Build history of the part. All positions in model axes, mm. Give positions to 0.01 mm unless a question says otherwise; leave off trailing zeros. Write each loop counter-clockwise with the first axis right and the second up, starting at its lowest first coordinate (ties: lowest second). Pieces come first, ordered by that corner, then holes. Notation, with made-up numbers: (-10, -8) -> (36, -8) arc R20 cw to (36, 16) -> close; hole circle Ø6 at (64.25, 70). An arc over 180 degrees is marked (long way). Write item = value, one per line. Start each with the question number.
Q1. Saw through at B-B, the plane y = 92.65. Give the number of separate pieces and of enclosed holes in the cut face, then the cut area to 3 significant figures.
Q2. Wall check: line 1 (X direction, y = 91.65, z = -6); line 2 (X direction, y = 92.9, z = -136.5); line 3 (X direction, y = 92.75, z = -112). Give the ranges that are in metal, low to high.
Q3. Drop a flat-ended pin along its axis: P1, Ø5, axis at x = 117, z = -6, coming from the +Y side. Give the stop position or say it passes through.
Q4. Saw through at A-A, the plane z = -21.5. List the corners of the cut face in (x, y), then the cut area to 3 significant figures.
from build123d import *

# Parameters (mm, degrees)
SKETCH1_W           = 123
SKETCH1_H           = 220
BOSS_EXTRUDE1_DEPTH = 4
SKETCH2_W           = 123
SKETCH2_H           = 220
SKETCH2_W_2         = 115
SKETCH2_H_2         = 212
BOSS_EXTRUDE2_DEPTH = 87
CUT_EXTRUDE1_REACH  = 269.974
SKETCH3_W           = 115
SKETCH3_H           = 45
CUT_EXTRUDE2_REACH  = 269.974
SKETCH4_W           = 150
SKETCH4_H           = 20
SKETCH6_W           = 24
SKETCH6_H           = 37
SKETCH6_R           = 1.45
BOSS_EXTRUDE4_DEPTH = 3
SKETCH8_W           = 12
SKETCH8_H           = 12
BOSS_EXTRUDE5_DEPTH = 10
CUT_EXTRUDE3_REACH  = 269.974
SKETCH9_R           = 1.95
CUT_EXTRUDE4_REACH  = 269.974
SKETCH10_W          = 99
SKETCH10_H          = 40
CHAMFER1_SIZE       = 10
BOSS_EXTRUDE6_START = 3
SKETCH11_W          = 123
SKETCH11_H          = 220
SKETCH11_R          = 1.95
BOSS_EXTRUDE6_DEPTH = 3
CHAMFER2_SIZE       = 2.05
SKETCH12_W          = 123
SKETCH12_H          = 91
CUT_EXTRUDE5_DEPTH  = 270.007434841
CHAMFER3_SIZE       = 2
CUT_EXTRUDE6_DEPTH  = 253.06745129


with BuildPart() as part:
    # Sketch1 → Boss-Extrude1 (new body)
    with BuildSketch(Plane(origin=(0, 0, 0), x_dir=(1, 0, 0), z_dir=(0, 1, 0))):
        with Locations((61.5, 110)):
            Rectangle(SKETCH1_W, SKETCH1_H)
    extrude(amount=BOSS_EXTRUDE1_DEPTH)

    # Sketch2 → Boss-Extrude2 (add)
    with BuildSketch(Plane(origin=(0, 4, 0), x_dir=(1, 0, 0), z_dir=(0, 1, 0))):
        with Locations((61.5, 110)):
            Rectangle(SKETCH2_W, SKETCH2_H)
        with Locations((61.5, 110)):
            Rectangle(SKETCH2_W_2, SKETCH2_H_2, mode=Mode.SUBTRACT)
    extrude(amount=BOSS_EXTRUDE2_DEPTH)

    # Sketch3 → Cut-Extrude1 (cut, up to next)
    with BuildSketch(Plane.XY, mode=Mode.PRIVATE) as cut_extrude1_sk1:
        with Locations((61.5, 26.5)):
            Rectangle(SKETCH3_W, SKETCH3_H)
    cut_extrude1_tool1 = extrude(cut_extrude1_sk1.sketch, amount=-CUT_EXTRUDE1_REACH, mode=Mode.PRIVATE) & part.part
    add(cut_extrude1_tool1.solids().sort_by_distance((61.5, 26.5, 0))[0], mode=Mode.SUBTRACT)

    # Sketch4 → Cut-Extrude2 (cut, up to next)
    with BuildSketch(Plane(origin=(123, 0, 0), x_dir=(0, 0, -1), z_dir=(1, 0, 0)), mode=Mode.PRIVATE) as cut_extrude2_sk1:
        with Locations((125, 81)):
            Rectangle(SKETCH4_W, SKETCH4_H)
    cut_extrude2_tool1 = extrude(cut_extrude2_sk1.sketch, amount=-CUT_EXTRUDE2_REACH, mode=Mode.PRIVATE) & part.part
    add(cut_extrude2_tool1.solids().sort_by_distance((123, 81, -125))[0], mode=Mode.SUBTRACT)

    # Sketch6 → Boss-Extrude4 (add)
    # profile 1 of 2: a face of its own
    with BuildSketch(Plane(origin=(0, 49, 0), x_dir=(-1, 0, 0), z_dir=(0, -1, 0))):
        with Locations((-16, 22.5)):
            Rectangle(SKETCH6_W, SKETCH6_H)
        with Locations(Location((-25, 27.5, 0), (0, 0, 90))):
            Circle(SKETCH6_R, mode=Mode.SUBTRACT)
        with Locations(Location((-25, 17.5, 0), (0, 0, 270))):
            Circle(SKETCH6_R, mode=Mode.SUBTRACT)
    # profile 2 of 2: a face of its own
    with BuildSketch(Plane(origin=(0, 49, 0), x_dir=(-1, 0, 0), z_dir=(0, -1, 0))):
        with Locations((-107, 22.5)):
            Rectangle(SKETCH6_W, SKETCH6_H)
        with Locations(Location((-98, 17.5, 0), (0, 0, 90))):
            Circle(SKETCH6_R, mode=Mode.SUBTRACT)
        with Locations(Location((-98, 27.5, 0), (0, 0, 270))):
            Circle(SKETCH6_R, mode=Mode.SUBTRACT)
    extrude(amount=-BOSS_EXTRUDE4_DEPTH)

    # Sketch8 → Boss-Extrude5 (add)
    with BuildSketch(Plane(origin=(0, 91, 0), x_dir=(1, 0, 0), z_dir=(0, 1, 0))):
        with Locations((117, 214)):
            Rectangle(SKETCH8_W, SKETCH8_H)
        with Locations((6, 214)):
            Rectangle(SKETCH8_W, SKETCH8_H)
        with Locations((117, 6)):
            Rectangle(SKETCH8_W, SKETCH8_H)
        with Locations((6, 6)):
            Rectangle(SKETCH8_W, SKETCH8_H)
    extrude(amount=-BOSS_EXTRUDE5_DEPTH)

    # Sketch9 → Cut-Extrude3 (cut, up to next)
    with BuildSketch(Plane(origin=(0, 91, 0), x_dir=(1, 0, 0), z_dir=(0, 1, 0)), mode=Mode.PRIVATE) as cut_extrude3_sk1:
        with Locations(Location((6, 214, 0), (0, 0, 270))):
            Circle(SKETCH9_R)
    cut_extrude3_tool1 = extrude(cut_extrude3_sk1.sketch, amount=-CUT_EXTRUDE3_REACH, mode=Mode.PRIVATE) & part.part
    # Sketch9 → Cut-Extrude3 (cut, up to next)
    with BuildSketch(Plane(origin=(0, 91, 0), x_dir=(1, 0, 0), z_dir=(0, 1, 0)), mode=Mode.PRIVATE) as cut_extrude3_sk2:
        with Locations(Location((117, 214, 0), (0, 0, 90))):
            Circle(SKETCH9_R)
    cut_extrude3_tool2 = extrude(cut_extrude3_sk2.sketch, amount=-CUT_EXTRUDE3_REACH, mode=Mode.PRIVATE) & part.part
    # Sketch9 → Cut-Extrude3 (cut, up to next)
    with BuildSketch(Plane(origin=(0, 91, 0), x_dir=(1, 0, 0), z_dir=(0, 1, 0)), mode=Mode.PRIVATE) as cut_extrude3_sk3:
        with Locations(Location((117, 6, 0), (0, 0, 270))):
            Circle(SKETCH9_R)
    cut_extrude3_tool3 = extrude(cut_extrude3_sk3.sketch, amount=-CUT_EXTRUDE3_REACH, mode=Mode.PRIVATE) & part.part
    # Sketch9 → Cut-Extrude3 (cut, up to next)
    with BuildSketch(Plane(origin=(0, 91, 0), x_dir=(1, 0, 0), z_dir=(0, 1, 0)), mode=Mode.PRIVATE) as cut_extrude3_sk4:
        with Locations(Location((6, 6, 0), (0, 0, 90))):
            Circle(SKETCH9_R)
    cut_extrude3_tool4 = extrude(cut_extrude3_sk4.sketch, amount=-CUT_EXTRUDE3_REACH, mode=Mode.PRIVATE) & part.part
    add(cut_extrude3_tool1.solids().sort_by_distance((6, 91, -214))[0], mode=Mode.SUBTRACT)
    add(cut_extrude3_tool2.solids().sort_by_distance((117, 91, -214))[0], mode=Mode.SUBTRACT)
    add(cut_extrude3_tool3.solids().sort_by_distance((117, 91, -6))[0], mode=Mode.SUBTRACT)
    add(cut_extrude3_tool4.solids().sort_by_distance((6, 91, -6))[0], mode=Mode.SUBTRACT)

    # Sketch10 → Cut-Extrude4 (cut, up to next)
    with BuildSketch(Plane(origin=(0, 0, -220), x_dir=(-1, 0, 0), z_dir=(0, 0, -1)), mode=Mode.PRIVATE) as cut_extrude4_sk1:
        with Locations((-61.5, 71)):
            Rectangle(SKETCH10_W, SKETCH10_H)
    cut_extrude4_tool1 = extrude(cut_extrude4_sk1.sketch, amount=-CUT_EXTRUDE4_REACH, mode=Mode.PRIVATE) & part.part
    add(cut_extrude4_tool1.solids().sort_by_distance((61.5, 71, -220))[0], mode=Mode.SUBTRACT)

    # Chamfer1
    chamfer1_edges = [part.edges().sort_by_distance(p)[0] for p in [
        (4, 52, -22.5),
        (119, 52, -22.5),
    ]]
    chamfer(chamfer1_edges, length=CHAMFER1_SIZE)

    # Sketch11 → Boss-Extrude6 (add)
    with BuildSketch(Plane(origin=(0, 91, 0), x_dir=(1, 0, 0), z_dir=(0, 1, 0)).offset(BOSS_EXTRUDE6_START)):
        with Locations((61.5, 110)):
            Rectangle(SKETCH11_W, SKETCH11_H)
        with Locations(Location((6, 214, 0), (0, 0, 270))):
            Circle(SKETCH11_R, mode=Mode.SUBTRACT)
        with Locations(Location((117, 214, 0), (0, 0, 270))):
            Circle(SKETCH11_R, mode=Mode.SUBTRACT)
        with Locations(Location((117, 6, 0), (0, 0, 270))):
            Circle(SKETCH11_R, mode=Mode.SUBTRACT)
        with Locations(Location((6, 6, 0), (0, 0, 270))):
            Circle(SKETCH11_R, mode=Mode.SUBTRACT)
    extrude(amount=-BOSS_EXTRUDE6_DEPTH)

    # Chamfer2
    chamfer2_edges = [part.edges().sort_by_distance(p)[0] for p in [
        (6, 94, -215.95),
        (117, 94, -215.95),
        (117, 94, -7.95),
        (6, 94, -7.95),
    ]]
    chamfer(chamfer2_edges, length=CHAMFER2_SIZE)

    # Sketch12 → Cut-Extrude5 (cut, through all)
    with BuildSketch(Plane(origin=(0, 0, -220), x_dir=(-1, 0, 0), z_dir=(0, 0, -1))):
        with Locations((-61.5, 45.5)):
            Rectangle(SKETCH12_W, SKETCH12_H)
    extrude(amount=-CUT_EXTRUDE5_DEPTH, mode=Mode.SUBTRACT)

    # Chamfer3
    chamfer3_edges = [part.edges().sort_by_distance(p)[0] for p in [
        (0, 94, -110),
        (61.5, 94, 0),
        (123, 94, -110),
        (61.5, 94, -220),
    ]]
    chamfer(chamfer3_edges, length=CHAMFER3_SIZE - 0.0001)  # a hair under: the kernel refuses the full size

    # Sketch13 → Cut-Extrude6 (cut, through all)
    with BuildSketch(Plane(origin=(0, 94, 0), x_dir=(1, 0, 0), z_dir=(0, 1, 0))):
        with BuildLine():
            Line((24.023340597, 150.305086528), (101.805086528, 72.523340597))
            ThreePointArc((101.805086528, 72.523340597), (101.805086528, 69.694913472), (98.976659403, 69.694913472))
            Line((98.976659403, 69.694913472), (21.194913472, 147.476659403))
            ThreePointArc((21.194913472, 147.476659403), (21.194913472, 150.305086528), (24.023340597, 150.305086528))
        make_face()
        with BuildLine():
            Line((24.023340597, 30.305086528), (41.805086528, 12.523340597))
            ThreePointArc((41.805086528, 12.523340597), (41.805086528, 9.694913472), (38.976659403, 9.694913472))
            Line((38.976659403, 9.694913472), (21.194913472, 27.476659403))
            ThreePointArc((21.194913472, 27.476659403), (21.194913472, 30.305086528), (24.023340597, 30.305086528))
        make_face()
        with BuildLine():
            Line((24.023340597, 50.305086528), (61.805086528, 12.523340597))
            ThreePointArc((61.805086528, 12.523340597), (61.805086528, 9.694913472), (58.976659403, 9.694913472))
            Line((58.976659403, 9.694913472), (21.194913472, 47.476659403))
            ThreePointArc((21.194913472, 47.476659403), (21.194913472, 50.305086528), (24.023340597, 50.305086528))
        make_face()
        with BuildLine():
            Line((24.023340597, 70.305086528), (81.805086528, 12.523340597))
            ThreePointArc((81.805086528, 12.523340597), (81.805086528, 9.694913472), (78.976659403, 9.694913472))
            Line((78.976659403, 9.694913472), (21.194913472, 67.476659403))
            ThreePointArc((21.194913472, 67.476659403), (21.194913472, 70.305086528), (24.023340597, 70.305086528))
        make_face()
        with BuildLine():
            Line((24.023340597, 90.305086528), (101.805086528, 12.523340597))
            ThreePointArc((101.805086528, 12.523340597), (101.805086528, 9.694913472), (98.976659403, 9.694913472))
            Line((98.976659403, 9.694913472), (21.194913472, 87.476659403))
            ThreePointArc((21.194913472, 87.476659403), (21.194913472, 90.305086528), (24.023340597, 90.305086528))
        make_face()
        with BuildLine():
            Line((24.023340597, 110.305086528), (101.805086528, 32.523340597))
            ThreePointArc((101.805086528, 32.523340597), (101.805086528, 29.694913472), (98.976659403, 29.694913472))
            Line((98.976659403, 29.694913472), (21.194913472, 107.476659403))
            ThreePointArc((21.194913472, 107.476659403), (21.194913472, 110.305086528), (24.023340597, 110.305086528))
        make_face()
        with BuildLine():
            Line((44.023340597, 210.305086528), (101.805086528, 152.523340597))
            ThreePointArc((101.805086528, 152.523340597), (101.805086528, 149.694913472), (98.976659403, 149.694913472))
            Line((98.976659403, 149.694913472), (41.194913472, 207.476659403))
            ThreePointArc((41.194913472, 207.476659403), (41.194913472, 210.305086528), (44.023340597, 210.305086528))
        make_face()
        with BuildLine():
            Line((24.023340597, 130.305086528), (101.805086528, 52.523340597))
            ThreePointArc((101.805086528, 52.523340597), (101.805086528, 49.694913472), (98.976659403, 49.694913472))
            Line((98.976659403, 49.694913472), (21.194913472, 127.476659403))
            ThreePointArc((21.194913472, 127.476659403), (21.194913472, 130.305086528), (24.023340597, 130.305086528))
        make_face()
        with BuildLine():
            Line((64.023340597, 210.305086528), (101.805086528, 172.523340597))
            ThreePointArc((101.805086528, 172.523340597), (101.805086528, 169.694913472), (98.976659403, 169.694913472))
            Line((98.976659403, 169.694913472), (61.194913472, 207.476659403))
            ThreePointArc((61.194913472, 207.476659403), (61.194913472, 210.305086528), (64.023340597, 210.305086528))
        make_face()
        with BuildLine():
            Line((24.023340597, 210.305086528), (101.805086528, 132.523340597))
            ThreePointArc((101.805086528, 132.523340597), (101.805086528, 129.694913472), (98.976659403, 129.694913472))
            Line((98.976659403, 129.694913472), (21.194913472, 207.476659403))
            ThreePointArc((21.194913472, 207.476659403), (21.194913472, 210.305086528), (24.023340597, 210.305086528))
        make_face()
        with BuildLine():
            Line((24.023340597, 190.305086528), (101.805086528, 112.523340597))
            ThreePointArc((101.805086528, 112.523340597), (101.805086528, 109.694913472), (98.976659403, 109.694913472))
            Line((98.976659403, 109.694913472), (21.194913472, 187.476659403))
            ThreePointArc((21.194913472, 187.476659403), (21.194913472, 190.305086528), (24.023340597, 190.305086528))
        make_face()
        with BuildLine():
            Line((24.023340597, 170.305086528), (101.805086528, 92.523340597))
            ThreePointArc((101.805086528, 92.523340597), (101.805086528, 89.694913472), (98.976659403, 89.694913472))
            Line((98.976659403, 89.694913472), (21.194913472, 167.476659403))
            ThreePointArc((21.194913472, 167.476659403), (21.194913472, 170.305086528), (24.023340597, 170.305086528))
        make_face()
        with BuildLine():
            Line((84.023340597, 210.305086528), (101.805086528, 192.523340597))
            ThreePointArc((101.805086528, 192.523340597), (101.805086528, 189.694913472), (98.976659403, 189.694913472))
            Line((98.976659403, 189.694913472), (81.194913472, 207.476659403))
            ThreePointArc((81.194913472, 207.476659403), (81.194913472, 210.305086528), (84.023340597, 210.305086528))
        make_face()
    extrude(amount=-CUT_EXTRUDE6_DEPTH, mode=Mode.SUBTRACT)


solid = part.part
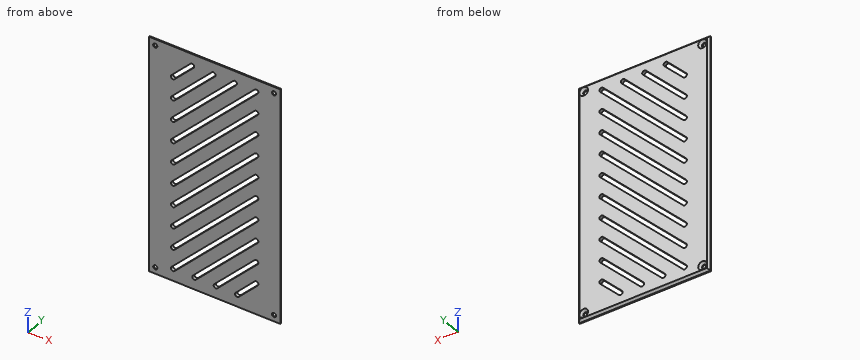
Report:
q1.separate_pieces = 1
q1.enclosed_holes = 17
q1.area = 22,000 mm2
q2.line_1 = 0 to 4.05, 7.95 to 115.05, 118.95 to 123
q2.line_2 = 0.9 to 32.17, 37.83 to 52.17, 57.83 to 72.17, 77.83 to 92.17, 97.83 to 122.1
q2.line_3 = 0.75 to 36.67, 42.33 to 56.67, 62.33 to 76.67, 82.33 to 96.67, 102.18 to 122.25
q3.P1 = 92.5
q4.outline = (0, 91) -> (27.17, 91) -> (27.17, 94) -> (2, 94) -> (0, 92) -> close; (32.83, 91) -> (47.17, 91) -> (47.17, 94) -> (32.83, 94) -> close; (52.83, 91) -> (67.17, 91) -> (67.17, 94) -> (52.83, 94) -> close; (72.83, 91) -> (87.17, 91) -> (87.17, 94) -> (72.83, 94) -> close; (92.83, 91) -> (123, 91) -> (123, 92) -> (121, 94) -> (92.83, 94) -> close
q4.area = 297 mm2
